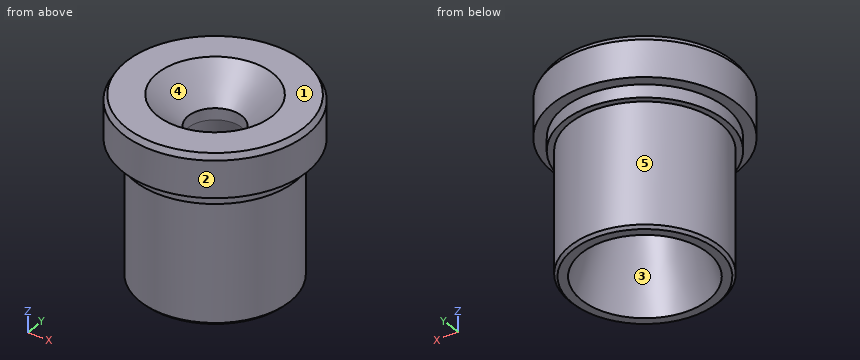
from build123d import *

# Parameters (mm, degrees)
CHAMFER1_SIZE  = 0.762
CHAMFER1_SIZE2 = 0.439940905
CHAMFER2_SIZE  = 0.381


with BuildPart() as part:
    # Sketch1 → Revolve1 (revolve)
    with BuildSketch(Plane(origin=(0, 0, 0), x_dir=(0, 0, -1), z_dir=(1, 0, 0)), mode=Mode.PRIVATE) as revolve1_sk:
        Polygon((24.638, -10.3251), (24.638, -8.7376), (5.821373033, -3.6957), (4.2418, -3.6957), (0, -7.9375), (0, -12.7), (5.842, -12.7), (5.842, -11.1633), (7.62, -11.1633), (7.62, -10.3251), align=None)
    revolve(revolve1_sk.sketch.rotate(Axis((0, 0, -6.716573557), (0, 0, -1)), 270), axis=Axis((0, 0, -6.716573557), (0, 0, -1)))

    # Chamfer1
    chamfer1_edges = [part.edges().sort_by_distance(p)[0] for p in [
        (-12.7, 0, 0),
    ]]
    chamfer1_side = [part.faces().sort_by_distance(p)[0] for p in [
        (-12.7, 0, -2.921),
    ]]
    chamfer(chamfer1_edges, length=CHAMFER1_SIZE, length2=CHAMFER1_SIZE2, reference=chamfer1_side[0])

    # Chamfer2
    chamfer2_edges = [part.edges().sort_by_distance(p)[0] for p in [
        (-10.3251, 0, -24.638),
    ]]
    chamfer(chamfer2_edges, length=CHAMFER2_SIZE)


solid = part.part
Geometry: final body of the model. Coordinates: model frame, mm. Face numbers are marked on the shaded views. A direction names the side the tool comes from. Give positions to 0.01 mm unless a question says otherwise; leave off trailing zeros. Write each loop counter-clockwise with the first axis right and the second up, starting at its lowest first coordinate (ties: lowest second). Pieces come first, ordered by that corner, then holes.
(1) Cut plane C-C, the plane z = -5. Return loops of the section in (x, y), then the cut area to 3 significant figures.
(2) Ray query, line 1 (Y direction, x = 0, z = -5.3); line 2 (Y direction, x = 0.75, z = -14.75); line 3 (X direction, y = -1, z = -17.25). Return the intervals inside material, ascending.
(3) Cut plane D-D, the plane z = -15.5. Return loops of the section in (x, y), then the cut area to 3 significant figures.
(4) Access query for the marked faces 4 and 5. Directions: +Z, -Z, +X, -X, +Y, -Y. A direction counts if a zero-diameter tool reaches every point of the face in a straight line with its end or side. Return the directions, or none.
(5) Cut plane A-A, the plane y = 0. Return loops of the section in (x, z).
(6) Mould query, pull axis X, two halves, no side actions, for the marked faces 1, 2 and 3. Classes: released by +X, released by -X, zero draft, split by the parting line, or undercut.
(7) First-contact query: P1, Ø2, axis at x = 9, y = 6, coming from the +Z side; P2, Ø12, axis at y = -5.5, z = -22, coming from the +X side; P3, Ø3, axis at y = 8, z = -20, coming from the -X side; P4, Ø10, axis at x = 1.5, z = -14.5, coming from the -Y side. Flat tips, straight axial feed; report the tip coordinate or a pass-through.
Values follow:
1. outline: circle Ø25.4 at (0, 0); hole circle Ø7.39 at (0, 0)
1. area: 464 mm2
2. line 1: y = -12.7 to -3.7, 3.7 to 12.7
2. line 2: y = -10.3 to -6.04, 6.04 to 10.3
2. line 3: x = -10.28 to -6.68, 6.68 to 10.28
3. outline: circle Ø20.65 at (0, 0); hole circle Ø12.58 at (0, 0)
3. area: 211 mm2
4. face 4: +Z
4. face 5: -Z
5. outline: (-12.7, -5.84) - (-11.16, -5.84) - (-11.16, -7.62) - (-10.33, -7.62) - (-10.33, -24.26) - (-9.94, -24.64) - (-8.74, -24.64) - (-3.7, -5.82) - (-3.7, -4.24) - (-7.94, 0) - (-12.26, 0) - (-12.7, -0.76) - close; (3.7, -5.82) - (8.74, -24.64) - (9.94, -24.64) - (10.33, -24.26) - (10.33, -7.62) - (11.16, -7.62) - (11.16, -5.84) - (12.7, -5.84) - (12.7, -0.76) - (12.26, 0) - (7.94, 0) - (3.7, -4.24) - close
6. face 1: zero draft
6. face 2: split by the parting line
6. face 3: undercut
7. P1: stops at z = 0
7. P2: stops at x = 10.33
7. P3: stops at x = -8.02
7. P4: stops at y = -10.33
